Source: CAD feature listing. Evaluate the final solid. Frame: model axes, mm. A direction names the side the tool comes from. Give positions to 0.01 mm unless a question says otherwise; leave off trailing zeros. Write each loop counter-clockwise with the first axis right and the second up, starting at its lowest first coordinate (ties: lowest second). Pieces come first, ordered by that corner, then holes. Notation, with made-up numbers: M 69.25,58.25 L 124.25,58.25 A25 ccw 124.25,77.25 Z; hole C 85,-35.75 d11. An arc over 180 degrees is marked long. Answer as a JSON object with one key per item and string values. Group by question number.
```python
from build123d import *

# Parameters (mm, degrees)
SKETCH7_R           = 102.108
SKETCH9_R           = 125.73
SKETCH11_R          = 102.108
BOSS_EXTRUDE1_DEPTH = 306.324
SKETCH12_R          = 125.73
BOSS_EXTRUDE2_DEPTH = 306.324


with BuildPart() as part:
    # Sketch7 → Loft3 section 0
    with BuildSketch(Plane(origin=(0, 0, 0), x_dir=(0, 0, -1), z_dir=(1, 0, 0))):
        Circle(SKETCH7_R)
    # Sketch9 → Loft3 section 1
    with BuildSketch(Plane(origin=(1021.373155762, 0, 0), x_dir=(0, 0, -1), z_dir=(1, 0, 0))):
        Circle(SKETCH9_R)
    loft()

    # Sketch11 → Boss-Extrude1 (add)
    with BuildSketch(Plane.ZY):
        with Locations(Location((0, 0, 0), (0, 0, 180))):
            Circle(SKETCH11_R)
    extrude(amount=BOSS_EXTRUDE1_DEPTH)

    # Sketch12 → Boss-Extrude2 (add)
    with BuildSketch(Plane(origin=(1021.373155762, 0, 0), x_dir=(0, 0, -1), z_dir=(1, 0, 0))):
        with Locations(Location((0, 0, 0), (0, 0, 180))):
            Circle(SKETCH12_R)
    extrude(amount=BOSS_EXTRUDE2_DEPTH)


solid = part.part
```
(1) Access query for faces 1 (the flat face through (1327.697, -2, -2)), 2 (the cylindrical face through (-151.018, -30.67, -97.393)). Directions: +Z, -Z, +X, -X, +Y, -Y. A direction counts if a zero-diameter tool reaches every point of the face in a straight line with its end or side. Return the directions, or none.
(2) Section A-A, the plane z = 0. Return loops of the section in (x, y), plus the area to 3 significant figures.
(3) Section B-B, the plane x = 1096.5. Return loops of the section in (y, z), plus the area to 3 significant figures.
(4) Contact query for flat-ended pins moving along their axis: pin 1 Ø5 at (x, z) = (72, -46) entering from -Y; pin 2 Ø2 at (x, y) = (-6, 30.5) entering from +Z; pin 3 Ø1 at (x, z) = (885.5, 11.5) entering from +Y. Output: stop coordinate, or through.
(5) Ray query, L1, parallel to Y at x = 356, z = -61; L2, parallel to Y at x = -220.5, z = -82; L3, parallel to Z at x = 1068, y = -11.5. Return the intervals inside material, ascending. Write a range as [from, to].
(6) Section C-C, the plane x = 272.5. Return loops of the section in (y, z), plus the area to 3 significant figures.
Reported:
{
 "1": {"face 1": "+Z, -Z, +X, +Y, -Y", "face 2": "-X"},
 "2": {"outline": "M -306.32,-102.11 L 0,-102.11 L 1021.37,-125.73 L 1327.7,-125.73 L 1327.7,125.73 L 1021.37,125.73 L 0,102.11 L -306.32,102.11 Z", "area": "372,000 mm2"},
 "3": {"outline": "C 0,0 d251.46", "area": "49,700 mm2"},
 "4": {"pin 1": "stops at y = -94.22", "pin 2": "stops at z = 97.75", "pin 3": "stops at y = 122.09"},
 "5": {"L1": "y = [-91.95, 91.95]", "L2": "y = [-60.84, 60.84]", "L3": "z = [-125.2, 125.2]"},
 "6": {"outline": "C 0,0 d216.82", "area": "36,900 mm2"}
}
